Can you work these out from the model? Positions are in its coordinate system, mm. A direction names the side the tool comes from. Give positions to 0.01 mm unless a question says otherwise; leave off trailing zeros. Write each loop counter-clockwise with the first axis right and the second up, starting at its lowest first coordinate (ties: lowest second). Pieces come first, ordered by that corner, then holes. Notation, with made-up numbers: (43, -37.75) - (75, -37.75) arc R18 cw to (75, -12.75) - close; hole circle Ø11 at (65, 39.5). An arc over 180 degrees is marked (long way). Use a Markdown table: item, result. Add a question column.
```python
from build123d import *

# Parameters (mm, degrees)
F1_DEPTH = 45
F2_R     = 6
F3_DEPTH = 30
F4_R     = 3
F5_DEPTH = 40.001


with BuildPart() as f1:
    # F0 (on Front) → F1 (new body)
    with BuildSketch(Plane.XZ):
        with BuildLine():
            Line((-43, 0), (0, 0))
            Line((0, 0), (0, 70))
            Line((0, 70), (-108, 70))
            Line((-108, 70), (-108, 0))
            Line((-108, 0), (-65, 0))
            ThreePointArc((-65, 0), (-54, 11), (-43, 0))
        make_face()
    extrude(amount=F1_DEPTH)

    # F2 (on face) → F3 (cut)
    with BuildSketch(Plane.XY.offset(70)):
        with Locations((-90, -12)):
            Circle(F2_R)
        with Locations((-90, -33)):
            Circle(F2_R)
        with Locations((-18, -12)):
            Circle(F2_R)
        with Locations((-18, -33)):
            Circle(F2_R)
    extrude(amount=-F3_DEPTH, mode=Mode.SUBTRACT)

    # F4 (on face) → F5 (cut, through all)
    with BuildSketch(Plane.XY.offset(40)):
        with Locations((-90, -12)):
            Circle(F4_R)
        with Locations((-18, -12)):
            Circle(F4_R)
        with Locations((-18, -33)):
            Circle(F4_R)
        with Locations((-90, -33)):
            Circle(F4_R)
    extrude(amount=-F5_DEPTH, mode=Mode.SUBTRACT)


solid = f1.part
```
Q1. If I drill on probe 1 along Y at (x, z) = (-18, 58.25); probe 2 along Y at (x, z) = (-18, 14); probe 3 along X at (y, z) = (-32, 28.5), over which ranges is the centre line in solid material (lowest first)? Write a range as [from, to].
Q2. If we mould it in two halves opening along X, with no side actions, what happens to faces 3 (the flat face through (-108, -22, 35)), 4 (the cylindrical face through (-96, -12, 55)), 5 (the cylindrical face through (-19.301, -38.857, 55.21)), 6 (the flat face through (-22, -22, 0))? For each: released by +X, released by -X, zero draft, split by the parting line, or undercut.
Q3. I'm going to push flat-ended pins straight in: P1, Ø2, axis at x = -13.5, y = -31, coming from the -Z side; P2, Ø3.5, axis at x = -88, y = -14.5, coming from the +Z side. Where does each tip first touch, or does it pass through?
Q4. Suppose I cut it at D-D (y = -2.5). Please give me the cut outline in (x, z).
Q5. Suppose I cut it at A-A (x = -18). Please give me the cut outline in (y, z).
Q6. On a 3-axis mill with a long thin cutter (end or side, diameter ignored), from which of +Z, -Z, +X, -X, +Y, -Y can I reach the whole of each face in a straight line? I mean faces 1 (the flat face through (-17, -9, 40)), 2 (the flat face through (0, -22, 35)). Say none if no direction works.
Q7. Suppose I cut it at C-C (z = 12.5). Please give me the cut outline in (x, y), and give its area (3 significant figures).
Q8. Suppose I cut it at B-B (y = -33). Please give me the cut outline in (x, z), and give its area (3 significant figures).
Derived:
| question | item | result |
|---|---|---|
| 1 | probe 1 | [-45, -39], [-27, -18], [-6, 0] |
| 1 | probe 2 | [-45, -36], [-30, -15], [-9, 0] |
| 1 | probe 3 | [-108, -92.83], [-87.17, -20.83], [-15.17, 0] |
| 2 | face 3 | released by -X |
| 2 | face 4 | undercut |
| 2 | face 5 | undercut |
| 2 | face 6 | zero draft |
| 3 | P1 | z = 0 |
| 3 | P2 | z = 40 |
| 4 | outline | (-108, 0) - (-65, 0) arc R11 cw to (-43, 0) - (0, 0) - (0, 70) - (-108, 70) - close |
| 5 | outline | (-45, 0) - (-36, 0) - (-36, 40) - (-39, 40) - (-39, 70) - (-45, 70) - close; (-30, 0) - (-15, 0) - (-15, 40) - (-18, 40) - (-18, 70) - (-27, 70) - (-27, 40) - (-30, 40) - close; (-9, 0) - (0, 0) - (0, 70) - (-6, 70) - (-6, 40) - (-9, 40) - close |
| 6 | face 1 | +Z |
| 6 | face 2 | +Z, -Z, +X, +Y, -Y |
| 7 | outline | (-108, -45) - (0, -45) - (0, 0) - (-108, 0) - close; hole circle Ø6 at (-90, -33); hole circle Ø6 at (-90, -12); hole circle Ø6 at (-18, -33); hole circle Ø6 at (-18, -12) |
| 7 | area | 4,750 mm² |
| 8 | outline | (-108, 0) - (-93, 0) - (-93, 40) - (-96, 40) - (-96, 70) - (-108, 70) - close; (-87, 0) - (-65, 0) arc R11 cw to (-43, 0) - (-21, 0) - (-21, 40) - (-24, 40) - (-24, 70) - (-84, 70) - (-84, 40) - (-87, 40) - close; (-15, 0) - (0, 0) - (0, 70) - (-12, 70) - (-12, 40) - (-15, 40) - close |
| 8 | area | 6,170 mm² |
